```python
from build123d import *

# Parameters (mm, degrees)
BOSS_EXTRUDE1_DEPTH = 80
CUT_EXTRUDE1_DEPTH  = 80
SKETCH3_W           = 20
SKETCH3_H           = 67.765549713
CUT_EXTRUDE2_DEPTH  = 15
SKETCH6_W           = 10
SKETCH6_H           = 40
CUT_EXTRUDE4_DEPTH  = 11


with BuildPart() as part:
    # Sketch1 → Boss-Extrude1 (new body)
    with BuildSketch(Plane.XY):
        Polygon((0, 50), (0, 0), (58, 0), (50, 20), (40, 20), (40, 50), align=None)
    extrude(amount=BOSS_EXTRUDE1_DEPTH)

    # Sketch2 → Cut-Extrude1 (cut)
    with BuildSketch(Plane.ZY):
        with BuildLine():
            Line((66.402636912, 50), (16.402636912, 50))
            ThreePointArc((16.402636912, 50), (41.402636912, 25), (66.402636912, 50))
        make_face()
    extrude(amount=-CUT_EXTRUDE1_DEPTH, mode=Mode.SUBTRACT)

    # Sketch3 → Cut-Extrude2 (cut)
    with BuildSketch(Plane(origin=(0, 50, 0), x_dir=(1, 0, 0), z_dir=(0, 1, 0))):
        with Locations((19.905264977, -39.117225144)):
            Rectangle(SKETCH3_W, SKETCH3_H)
    extrude(amount=-CUT_EXTRUDE2_DEPTH, mode=Mode.SUBTRACT)

    # Sketch6 → Cut-Extrude4 (cut)
    with BuildSketch(Plane(origin=(0, 20, 0), x_dir=(1, 0, 0), z_dir=(0, 1, 0))):
        with Locations((50, -40)):
            Rectangle(SKETCH6_W, SKETCH6_H)
    extrude(amount=-CUT_EXTRUDE4_DEPTH, mode=Mode.SUBTRACT)


solid = part.part
```
Geometry: final body of the model. Coordinates: model frame, mm. A direction names the side the tool comes from. Coordinates: 2 decimals unless noted, no trailing zeros. Loops run counter-clockwise (first coordinate to the right, second up) from the corner with the lowest first, then second, coordinate; pieces in that order, holes last. Notation, with made-up numbers: (29.25, 75.5) -> (62.25, 75.5) arc R22 ccw to (62.25, 107.5) -> close; hole circle Ø2 at (-15, -3). An arc over 180 degrees is marked (long way). Use a Markdown table: item, result. Add a question column.
(1) Section query C-C, the plane y = 38.5. Return loops of the section in (x, z), plus the area to 3 significant figures.
(2) Section query B-B, the plane z = 9.5. Return loops of the section in (x, y), plus the area to 3 significant figures.
(3) Mould query, pull axis Z, two halves, no side actions, for faces 1 (the cylindrical face through (19.72, 25.006, 40.853)), 2 (the flat face through (22, 25, 80)), 3 (the flat face through (40, 24.8, 39.4)). Classes: pulls with the +Z half, pulls with the -Z half, needs draft (parallel to the pull), parting line crosses it, or undercut.
(4) Section query D-D, the plane x = 25. Return loops of the section in (y, z), plus the area to 3 significant figures.
(5) Line query: line 1 along Z through (x, y) = (23, 44); line 2 along Y through (x, z) = (46, 66); line 3 along Y through (x, z) = (13, 5.5). Output: solid intervals per line, ascending.
(6) Access query for faces 4 (the flat face through (49, 15, 20)), 5 (the flat face through (9.905, 41, 69)), 6 (the flat face through (44, 20, 39)). Directions: +Z, -Z, +X, -X, +Y, -Y. A direction counts if a zero-diameter tool reaches every point of the face in a straight line with its end or side. Return the directions, or none.
(7) Section query A-A, the plane y = 11.5. Return loops of the section in (x, z), plus the area to 3 significant figures.
(8) Pin query (flat end, axial travel): pin 1 Ø12 at (y, z) = (18.5, 42) entering from -X; pin 2 Ø6 at (y, z) = (44, 67) entering from +X; pin 3 Ø6 at (y, z) = (9, 52.5) entering from +X; pin 4 Ø10.5 at (x, z) = (48.5, 42.5) entering from +Y. Return the tip coordinate at first contact, or that it passes through.
Answer:
| question | item | result |
|---|---|---|
| 1 | outline | (0, 0) -> (40, 0) -> (40, 19.2) -> (29.91, 19.2) -> (29.91, 5.23) -> (9.91, 5.23) -> (9.91, 19.2) -> (0, 19.2) -> close; (0, 63.6) -> (9.91, 63.6) -> (9.91, 73) -> (29.91, 73) -> (29.91, 63.6) -> (40, 63.6) -> (40, 80) -> (0, 80) -> close |
| 1 | area | 957 mm^2 |
| 2 | outline | (0, 0) -> (58, 0) -> (50, 20) -> (40, 20) -> (40, 50) -> (29.91, 50) -> (29.91, 35) -> (9.91, 35) -> (9.91, 50) -> (0, 50) -> close |
| 2 | area | 1,980 mm^2 |
| 3 | face 1 | undercut |
| 3 | face 2 | pulls with the +Z half |
| 3 | face 3 | needs draft |
| 4 | outline | (0, 0) -> (50, 0) -> (50, 5.23) -> (35, 5.23) -> (35, 21.4) arc R25 cw to (35, 61.4) -> (35, 73) -> (50, 73) -> (50, 80) -> (0, 80) -> close |
| 4 | area | 2,700 mm^2 |
| 5 | line 1 | z = 0 to 5.23, 73 to 80 |
| 5 | line 2 | y = 0 to 20 |
| 5 | line 3 | y = 0 to 35 |
| 6 | face 4 | +X, +Y |
| 6 | face 5 | +Y |
| 6 | face 6 | +Z, -Z, +X, +Y |
| 7 | outline | (0, 0) -> (53.4, 0) -> (53.4, 20) -> (45, 20) -> (45, 60) -> (53.4, 60) -> (53.4, 80) -> (0, 80) -> close |
| 7 | area | 3,940 mm^2 |
| 8 | pin 1 | stops at x = 0 |
| 8 | pin 2 | stops at x = 40 |
| 8 | pin 3 | stops at x = 55.6 |
| 8 | pin 4 | stops at y = 20 |
